Geometry check sheet. Reference: the model listing, model coordinates, mm. Face numbers are marked on the shaded views. A direction names the side the tool comes from. Coordinates: 2 decimals unless noted, no trailing zeros. Write each loop counter-clockwise with the first axis right and the second up, starting at its lowest first coordinate (ties: lowest second). Pieces come first, ordered by that corner, then holes. Notation, with made-up numbers: (37, 58) - (63, 58) arc R22 cw to (63, 73) - close; hole circle Ø8 at (-13, 27.25). An arc over 180 degrees is marked (long way). Answer as a JSON object with one key per item and string values. Group by question number.
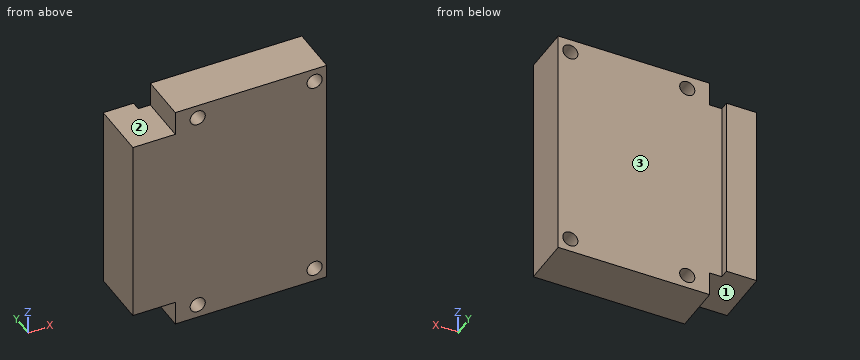
from build123d import *

# Parameters (mm, degrees)
SKETCH_2_R      = 2.5
EXTRUDE_2_DEPTH = 16
SKETCH_5_W      = 10
SKETCH_5_H      = 62
EXTRUDE_3_DEPTH = 3


with BuildPart() as part:
    # 草图2 → 凸台-拉伸2 (new body)
    with BuildSketch(Plane(origin=(0, 0, 0), x_dir=(1, 0, 0), z_dir=(0, 1, 0))):
        Polygon((-18, 39), (-18, 31), (-32, 31), (-32, -31), (-18, -31), (-18, -39), (32, -39), (32, 39), align=None)
        with Locations(Location((28, 34.5, 0), (0, 0, 270))):
            Circle(SKETCH_2_R, mode=Mode.SUBTRACT)
        with Locations(Location((-10.6, 34.5, 0), (0, 0, 270))):
            Circle(SKETCH_2_R, mode=Mode.SUBTRACT)
        with Locations(Location((28, -34.5, 0), (0, 0, 270))):
            Circle(SKETCH_2_R, mode=Mode.SUBTRACT)
        with Locations(Location((-10.6, -34.5, 0), (0, 0, 270))):
            Circle(SKETCH_2_R, mode=Mode.SUBTRACT)
    extrude(amount=EXTRUDE_2_DEPTH)

    # 草图5 → 凸台-拉伸3 (add)
    with BuildSketch(Plane(origin=(0, 16, 0), x_dir=(1, 0, 0), z_dir=(0, 1, 0))):
        with Locations((-27, 0)):
            Rectangle(SKETCH_5_W, SKETCH_5_H)
    extrude(amount=EXTRUDE_3_DEPTH)


solid = part.part
(1) Section check D-D (z = 4.5). Record the cut outline in (x, y).
(2) Section check B-B (x = -10.6). Record the cut outline in (y, z), and give its area (3 significant figures).
(3) Set-up check for the marked faces 1, 2 and 3: record each of +Z, -Z, +X, -X, +Y, -Y from which the full face is reachable in a straight line by a thin tool's end or side.
(4) Section check A-A (y = 7.5). Record the cut outline in (x, z), and give its area (3 significant figures).
(5) Section check C-C (z = -34.5). Record the cut outline in (x, y).
(6) Gauge pin test, flat ends, axial feed: pin 1 (6 mm diameter, centred on x = -10.6, z = 34.5, fed in from +Y); pin 2 (4 mm diameter, centred on y = 6, z = 35.5, fed in from -X); pin 3 (11 mm diameter, centred on x = -28.5, y = 13.5, fed in from -Z). Record the tip position at first contact, or that the pin passes through.
(7) Material ranges on L1, parallel to X at y = 6.5, z = -34.5; L2, parallel to Y at x = 19, z = 25.5; L3, parallel to X at y = 16.5, z = 5.5, recorded low to high. Write a range as [from, to].
Conclusion:
{
 "1": {"outline": "(-32, 0) - (32, 0) - (32, 16) - (-22, 16) - (-22, 19) - (-32, 19) - close"},
 "2": {"outline": "(0, -39) - (16, -39) - (16, -37) - (0, -37) - close; (0, -32) - (16, -32) - (16, 32) - (0, 32) - close; (0, 37) - (16, 37) - (16, 39) - (0, 39) - close", "area": "1,090 mm^2"},
 "3": {"face 1": "-Z, -X, +Y, -Y", "face 2": "+Z, -X, +Y, -Y", "face 3": "+Z, -Z, +X, +Y"},
 "4": {"outline": "(-32, -31) - (-18, -31) - (-18, -39) - (32, -39) - (32, 39) - (-18, 39) - (-18, 31) - (-32, 31) - close; hole circle Ø5 at (-10.6, -34.5); hole circle Ø5 at (-10.6, 34.5); hole circle Ø5 at (28, -34.5); hole circle Ø5 at (28, 34.5)", "area": "4,690 mm^2"},
 "5": {"outline": "(-18, 0) - (-13.1, 0) - (-13.1, 16) - (-18, 16) - close; (-8.1, 0) - (25.5, 0) - (25.5, 16) - (-8.1, 16) - close; (30.5, 0) - (32, 0) - (32, 16) - (30.5, 16) - close"},
 "6": {"pin 1": "stops at y = 16", "pin 2": "stops at x = -18", "pin 3": "stops at z = -31"},
 "7": {"L1": "x = [-18, -13.1], [-8.1, 25.5], [30.5, 32]", "L2": "y = [0, 16]", "L3": "x = [-32, -22]"}
}
